Check sheet for the modelled part. Datum: model origin and axes. Units: mm. A direction names the side the tool comes from. Round coordinates to 2 decimals unless told otherwise and drop trailing zeros. Loops run counter-clockwise (first coordinate to the right, second up) from the corner with the lowest first, then second, coordinate; pieces in that order, holes last. Notation, with made-up numbers: M 51,79.25 L 107,79.25 A17 ccw 107,95.25 Z; hole C 68,-24.75 d8. An arc over 180 degrees is marked long. One line per question, with ' | ' between items. Start each with the question number.
(1) Section check A-A (y = 0). Record the boundary of the cut face in (x, z).
(2) Tool access check on faces 4 (the face through (7, 0, 6)), 5 (the face through (-6.459, 8.087, 5.972)), 6 (the face through (0, -7, 6)), 7 (the face through (7.282, 7.355, 5.972)). Record the directions out of +Z, -Z, +X, -X, +Y, -Y that give a thin tool (end or side, any length) a straight path to the whole face; none if there is none.
(3) Section check C-C (y = -12). Record the boundary of the cut face in (x, z), and give its area (3 significant figures).
(4) Draft check along Y on faces 1 (the face through (-7.282, -7.355, 5.972)), 2 (the face through (9.5, -0.1, 2)), 3 (the face through (-8.356, 6.108, 5.972)). Enter one of: +Y half, -Y half, draft (parallel to the pull), parting line (faces both ways), or undercut.
(5) Thickness scan on probe 1 along Y at (x, z) = (0, 5); probe 2 along Y at (x, z) = (0, 3); probe 3 along X at (y, z) = (6, 5.5). Record the ranges inside material, lowest first. Write a range as [from, to].
(6) Go/stop test with flat-tipped pins: P1, Ø2, axis at y = 7.5, z = 2.5, coming from the +X side; P2, Ø4.5, axis at x = -12, y = 0, coming from the +Z side; P3, Ø10, axis at x = 10.5, y = 9, coming from the -Z side; P4, Ø2, axis at y = -10, z = 6, coming from the +X side. Record where each tip stops, or that it passes through.
(7) Section check D-D (z = 2.25). Count the separate pieces of the cut face and the enclosed holes in it, and give its area (3 significant figures).
(8) Section check B-B (x = 2). Record the boundary of the cut face in (y, z).
Autodesk Inventor part; units mm, degrees
ref_plane "YZ Plane" through (0, 0, 0) normal (1, 0, 0) x (0, 1, 0)
ref_plane "XZ Plane" through (0, 0, 0) normal (0, 1, 0) x (-1, 0, 0)
ref_plane "XY Plane" through (0, 0, 0) normal (0, 0, 1) x (1, 0, 0)
sketch "Sketch1" plane through (0, 0, 0) normal (0, 0, 1) x (1, 0, 0)
  circle A0 centre (0, 0) radius 16
  circle A1 centre (0, 0) radius 4
  circle A2 centre (12, 0) radius 2.5
  circle A3 centre (0, 12) radius 2.5
  circle A4 centre (-12, 0) radius 2.5
  circle A5 centre (0, -12) radius 2.5
  dimension "d0" = 32
  dimension "d1" = 8
  dimension "d2" = 5
  dimension "d3" = 12
  dimension "d6" = 360
extrude "Extrusion1" add sketch "Sketch1" along normal blind 4 contours A0 | A1
sketch "Sketch3" plane through (0, 0, 4) normal (0, 0, 1) x (1, 0, 0)
  arc A0 (-6.9584, 12.5904) -> (-5.9892, 8.4411) centre (5.202, 13.243) ccw
  arc A1 (-5.9892, 8.4411) -> (-6.8967, 7.7174) centre (0, 0) ccw
  arc A2 (-6.8967, 7.7174) -> (-10.7263, 9.5856) centre (-14.0685, -2.1247) ccw
  arc A3 (-10.7263, 9.5856) -> (-11.7321, 8.3244) centre (0, 0) ccw
  arc A4 (-11.7321, 8.3244) -> (-9.0586, 5.0065) centre (-1.0591, 14.1885) ccw
  arc A5 (-9.0586, 5.0065) -> (-9.5622, 3.9608) centre (0, 0) ccw
  arc A6 (-9.5622, 3.9608) -> (-13.8231, 3.9824) centre (-11.7534, -8.0184) ccw
  arc A7 (-13.8231, 3.9824) -> (-14.1821, 2.4096) centre (0, 0) ccw
  arc A8 (-14.1821, 2.4096) -> (-10.3337, 0.5803) centre (-7.1104, 12.3239) ccw
  arc A9 (-10.3337, 0.5803) -> (-10.3337, -0.5803) centre (0, 0) ccw
  arc A10 (-10.3337, -0.5803) -> (-14.1821, -2.4096) centre (-7.1104, -12.3239) ccw
  arc A11 (-14.1821, -2.4096) -> (-13.8231, -3.9824) centre (0, 0) ccw
  arc A12 (-13.8231, -3.9824) -> (-9.5622, -3.9608) centre (-11.7534, 8.0184) ccw
  arc A13 (-9.5622, -3.9608) -> (-9.0586, -5.0065) centre (0, 0) ccw
  arc A14 (-9.0586, -5.0065) -> (-11.7321, -8.3244) centre (-1.0591, -14.1885) ccw
  arc A15 (-11.7321, -8.3244) -> (-10.7263, -9.5856) centre (0, 0) ccw
  arc A16 (-10.7263, -9.5856) -> (-6.8967, -7.7174) centre (-14.0685, 2.1247) ccw
  arc A17 (-6.8967, -7.7174) -> (-5.9892, -8.4411) centre (0, 0) ccw
  arc A18 (-5.9892, -8.4411) -> (-6.9584, -12.5904) centre (5.202, -13.243) ccw
  arc A19 (-6.9584, -12.5904) -> (-5.505, -13.2903) centre (0, 0) ccw
  arc A20 (-5.505, -13.2903) -> (-2.8652, -9.9455) centre (-13.5971, -4.1898) ccw
  arc A21 (-2.8652, -9.9455) -> (-1.7337, -10.2038) centre (0, 0) ccw
  arc A22 (-1.7337, -10.2038) -> (-0.8066, -14.3627) centre (10.4327, -9.6744) ccw
  arc A23 (-0.8066, -14.3627) -> (0.8066, -14.3627) centre (0, 0) ccw
  arc A24 (0.8066, -14.3627) -> (1.7337, -10.2038) centre (-10.4327, -9.6744) ccw
  arc A25 (1.7337, -10.2038) -> (2.8652, -9.9455) centre (0, 0) ccw
  arc A26 (2.8652, -9.9455) -> (5.505, -13.2903) centre (13.5971, -4.1898) ccw
  arc A27 (5.505, -13.2903) -> (6.9584, -12.5904) centre (0, 0) ccw
  arc A28 (6.9584, -12.5904) -> (5.9892, -8.4411) centre (-5.202, -13.243) ccw
  arc A29 (5.9892, -8.4411) -> (6.8967, -7.7174) centre (0, 0) ccw
  arc A30 (6.8967, -7.7174) -> (10.7263, -9.5856) centre (14.0685, 2.1247) ccw
  arc A31 (10.7263, -9.5856) -> (11.7321, -8.3244) centre (0, 0) ccw
  arc A32 (11.7321, -8.3244) -> (9.0586, -5.0065) centre (1.0591, -14.1885) ccw
  arc A33 (9.0586, -5.0065) -> (9.5622, -3.9608) centre (0, 0) ccw
  arc A34 (9.5622, -3.9608) -> (13.8231, -3.9824) centre (11.7534, 8.0184) ccw
  arc A35 (13.8231, -3.9824) -> (14.1821, -2.4096) centre (0, 0) ccw
  arc A36 (14.1821, -2.4096) -> (10.3337, -0.5803) centre (7.1104, -12.3239) ccw
  arc A37 (10.3337, -0.5803) -> (10.3337, 0.5803) centre (0, 0) ccw
  arc A38 (10.3337, 0.5803) -> (14.1821, 2.4096) centre (7.1104, 12.3239) ccw
  arc A39 (14.1821, 2.4096) -> (13.8231, 3.9824) centre (0, 0) ccw
  arc A40 (13.8231, 3.9824) -> (9.5622, 3.9608) centre (11.7534, -8.0184) ccw
  arc A41 (9.5622, 3.9608) -> (9.0586, 5.0065) centre (0, 0) ccw
  arc A42 (9.0586, 5.0065) -> (11.7321, 8.3244) centre (1.0591, 14.1885) ccw
  arc A43 (11.7321, 8.3244) -> (10.7263, 9.5856) centre (0, 0) ccw
  arc A44 (10.7263, 9.5856) -> (6.8967, 7.7174) centre (14.0685, -2.1247) ccw
  arc A45 (6.8967, 7.7174) -> (5.9892, 8.4411) centre (0, 0) ccw
  arc A46 (5.9892, 8.4411) -> (6.9584, 12.5904) centre (-5.202, 13.243) ccw
  arc A47 (6.9584, 12.5904) -> (5.505, 13.2903) centre (0, 0) ccw
  arc A48 (5.505, 13.2903) -> (2.8652, 9.9455) centre (13.5971, 4.1898) ccw
  arc A49 (2.8652, 9.9455) -> (1.7337, 10.2038) centre (0, 0) ccw
  arc A50 (1.7337, 10.2038) -> (0.8066, 14.3627) centre (-10.4327, 9.6744) ccw
  arc A51 (0.8066, 14.3627) -> (-0.8066, 14.3627) centre (0, 0) ccw
  arc A52 (-0.8066, 14.3627) -> (-1.7337, 10.2038) centre (10.4327, 9.6744) ccw
  arc A53 (-1.7337, 10.2038) -> (-2.8652, 9.9455) centre (0, 0) ccw
  arc A54 (-2.8652, 9.9455) -> (-5.505, 13.2903) centre (-13.5971, 4.1898) ccw
  arc A55 (-5.505, 13.2903) -> (-6.9584, 12.5904) centre (0, 0) ccw
extrude "Extrusion3" add sketch "Sketch3" along normal blind 4
sketch "Sketch2" plane through (0, 0, 4) normal (0, 0, 1) x (1, 0, 0)
  circle A0 centre (12, 0) radius 2.5
  arc A1 (-1.7381, -10.203) -> (1.7381, -10.203) centre (0, -12) ccw
  arc A2 (1.7381, 10.203) -> (-1.7381, 10.203) centre (0, 12) ccw
  arc A3 (13.5312, -1.9762) -> (13.5312, 1.9762) centre (12, 0) ccw
  circle A4 centre (0, 0) radius 16 construction
  circle A5 centre (12, 0) radius 4.5
  circle A6 centre (0, 12) radius 4.5
  circle A7 centre (-12, 0) radius 4.5
  circle A8 centre (0, -12) radius 4.5
  arc A9 (14.1821, -2.4096) -> (13.5312, -1.9762) centre (7.1104, -12.3239) ccw
  arc A10 (13.8231, -3.9824) -> (14.1821, -2.4096) centre (0, 0) ccw
  arc A11 (9.5622, -3.9608) -> (13.8231, -3.9824) centre (11.7534, 8.0184) ccw
  arc A12 (9.0586, -5.0065) -> (9.5622, -3.9608) centre (0, 0) ccw
  arc A13 (11.7321, -8.3244) -> (9.0586, -5.0065) centre (1.0591, -14.1885) ccw
  arc A14 (10.7263, -9.5856) -> (11.7321, -8.3244) centre (0, 0) ccw
  arc A15 (6.8967, -7.7174) -> (10.7263, -9.5856) centre (14.0685, 2.1247) ccw
  arc A16 (5.9892, -8.4411) -> (6.8967, -7.7174) centre (0, 0) ccw
  arc A17 (6.9584, -12.5904) -> (5.9892, -8.4411) centre (-5.202, -13.243) ccw
  arc A18 (5.505, -13.2903) -> (6.9584, -12.5904) centre (0, 0) ccw
  arc A19 (2.8652, -9.9455) -> (5.505, -13.2903) centre (13.5971, -4.1898) ccw
  arc A20 (1.7381, -10.203) -> (2.8652, -9.9455) centre (0, 0) ccw
  arc A21 (-2.8652, -9.9455) -> (-1.7381, -10.203) centre (0, 0) ccw
  arc A22 (-5.505, -13.2903) -> (-2.8652, -9.9455) centre (-13.5971, -4.1898) ccw
  arc A23 (-6.9584, -12.5904) -> (-5.505, -13.2903) centre (0, 0) ccw
  arc A24 (-5.9892, -8.4411) -> (-6.9584, -12.5904) centre (5.202, -13.243) ccw
  arc A25 (-6.8967, -7.7174) -> (-5.9892, -8.4411) centre (0, 0) ccw
  arc A26 (-10.7263, -9.5856) -> (-6.8967, -7.7174) centre (-14.0685, 2.1247) ccw
  arc A27 (-11.7321, -8.3244) -> (-10.7263, -9.5856) centre (0, 0) ccw
  arc A28 (-9.0586, -5.0065) -> (-11.7321, -8.3244) centre (-1.0591, -14.1885) ccw
  arc A29 (-9.5622, -3.9608) -> (-9.0586, -5.0065) centre (0, 0) ccw
  arc A30 (-13.8231, -3.9824) -> (-9.5622, -3.9608) centre (-11.7534, 8.0184) ccw
  arc A31 (-14.1821, -2.4096) -> (-13.8231, -3.9824) centre (0, 0) ccw
  arc A32 (-13.5312, -1.9762) -> (-14.1821, -2.4096) centre (-7.1104, -12.3239) ccw
  arc A33 (-13.5312, 1.9762) -> (-13.5312, -1.9762) centre (-12, 0) ccw
  arc A34 (-14.1821, 2.4096) -> (-13.5312, 1.9762) centre (-7.1104, 12.3239) ccw
  arc A35 (-13.8231, 3.9824) -> (-14.1821, 2.4096) centre (0, 0) ccw
  arc A36 (-9.5622, 3.9608) -> (-13.8231, 3.9824) centre (-11.7534, -8.0184) ccw
  arc A37 (-9.0586, 5.0065) -> (-9.5622, 3.9608) centre (0, 0) ccw
  arc A38 (-11.7321, 8.3244) -> (-9.0586, 5.0065) centre (-1.0591, 14.1885) ccw
  arc A39 (-10.7263, 9.5856) -> (-11.7321, 8.3244) centre (0, 0) ccw
  arc A40 (-6.8967, 7.7174) -> (-10.7263, 9.5856) centre (-14.0685, -2.1247) ccw
  arc A41 (-5.9892, 8.4411) -> (-6.8967, 7.7174) centre (0, 0) ccw
  arc A42 (-6.9584, 12.5904) -> (-5.9892, 8.4411) centre (5.202, 13.243) ccw
  arc A43 (-5.505, 13.2903) -> (-6.9584, 12.5904) centre (0, 0) ccw
  arc A44 (-2.8652, 9.9455) -> (-5.505, 13.2903) centre (-13.5971, 4.1898) ccw
  arc A45 (-1.7381, 10.203) -> (-2.8652, 9.9455) centre (0, 0) ccw
  arc A46 (2.8652, 9.9455) -> (1.7381, 10.203) centre (0, 0) ccw
  arc A47 (5.505, 13.2903) -> (2.8652, 9.9455) centre (13.5971, 4.1898) ccw
  arc A48 (6.9584, 12.5904) -> (5.505, 13.2903) centre (0, 0) ccw
  arc A49 (5.9892, 8.4411) -> (6.9584, 12.5904) centre (-5.202, 13.243) ccw
  arc A50 (6.8967, 7.7174) -> (5.9892, 8.4411) centre (0, 0) ccw
  arc A51 (10.7263, 9.5856) -> (6.8967, 7.7174) centre (14.0685, -2.1247) ccw
  arc A52 (11.7321, 8.3244) -> (10.7263, 9.5856) centre (0, 0) ccw
  arc A53 (9.0586, 5.0065) -> (11.7321, 8.3244) centre (1.0591, 14.1885) ccw
  arc A54 (9.5622, 3.9608) -> (9.0586, 5.0065) centre (0, 0) ccw
  arc A55 (13.8231, 3.9824) -> (9.5622, 3.9608) centre (11.7534, -8.0184) ccw
  arc A56 (14.1821, 2.4096) -> (13.8231, 3.9824) centre (0, 0) ccw
  arc A57 (13.5312, 1.9762) -> (14.1821, 2.4096) centre (7.1104, 12.3239) ccw
  dimension "d10" = 9
  dimension "d13" = 360
extrude "Extrusion4" cut sketch "Sketch2" along normal blind 4 contours A0 | A0 A57 A56 A55 A5 A11 A10 A9 | A0 A9 A10 A11 A5 A55 A56 A57 | A47 A46 A2 A45 A44 A6 | A6 A44 A45 A2 A46 A47 | A19 A20 A1 A21 A22 A8 | A8 A22 A21 A1 A20 A19 | A36 A35 A34 A33 A32 A31 A30 A7 | A7 A30 A31 A32 A33 A34 A35 A36
sketch "Sketch4" plane through (0, 0, 8) normal (0, 0, 1) x (1, 0, 0)
  circle A0 centre (5, 0) radius 0.85
  circle A1 centre (0, 5) radius 0.85
  circle A2 centre (-5, 0) radius 0.85
  circle A3 centre (0, -5) radius 0.85
  circle A4 centre (5.6569, 5.6569) radius 0.85
  line L0 (0, 0) -> (5.6569, 5.6569) construction
  line L1 (0, 0) -> (5, 0) construction
  circle A5 centre (-5.6569, 5.6569) radius 0.85
  circle A6 centre (-5.6569, -5.6569) radius 0.85
  circle A7 centre (5.6569, -5.6569) radius 0.85
  circle A8 centre (0, 0) radius 0.85
  dimension "d21" = 1.7
  dimension "d22" = 5
  dimension "d25" = 360
  dimension "d27" = 1.7
  dimension "d28" = 45
  dimension "d29" = 8
  dimension "d32" = 360
  dimension "d34" = 1.7
extrude "Extrusion5" cut sketch "Sketch4" against normal through all
sketch "Sketch5" plane through (0, 0, 4) normal (0, 0, 1) x (1, 0, 0)
  circle A0 centre (0, 0) radius 0.85
  arc A1 (-5.9892, 8.4411) -> (-6.8967, 7.7174) centre (0, 0) ccw
  circle A2 centre (0, 0) radius 10.35
  circle A3 centre (0, 0) radius 16
extrude "Extrusion6" cut sketch "Sketch5" along normal through all contours A3
sketch "Sketch6" plane through (0, 0, 4) normal (0, 0, 1) x (1, 0, 0)
  circle A0 centre (12, 0) radius 2.5
  circle A1 centre (12, 0) radius 5
  circle A2 centre (0, 12) radius 5
  circle A3 centre (-12, 0) radius 5
  circle A4 centre (0, -12) radius 5
  point P0 (0, 0)
  dimension "d39" = 10
  dimension "d42" = 360
extrude "Extrusion7" cut sketch "Sketch6" along normal through all contours A0 | A1 | A2 | A3 | A4
properties part number "AC08" material "ABS Plastic"
The answers:
1) outline: M -16,0 L -14.5,0 L -14.5,4 L -16,4 Z; M -9.5,0 L -5.85,0 L -5.85,8 L -7,8 L -7,4 L -9.5,4 Z; M -4.15,0 L -0.85,0 L -0.85,8 L -4.15,8 Z; M 0.85,0 L 4.15,0 L 4.15,8 L 0.85,8 Z; M 5.85,0 L 9.5,0 L 9.5,4 L 7,4 L 7,8 L 5.85,8 Z; M 14.5,0 L 16,0 L 16,4 L 14.5,4 Z
2) face 4: +Z, +X | face 5: +Z, -X, +Y | face 6: +Z, -Y | face 7: +Z, +X, +Y
3) outline: M -10.58,0 L -2.5,0 L -2.5,4 L -10.58,4 Z; M 2.5,0 L 10.58,0 L 10.58,4 L 2.5,4 Z | area: 64.7 mm²
4) face 1: -Y half | face 2: undercut | face 3: +Y half
5) probe 1: [-7, -5.85], [-4.15, -0.85], [0.85, 4.15], [5.85, 7] | probe 2: [-16, -14.5], [-9.5, -5.85], [-4.15, -0.85], [0.85, 4.15], [5.85, 9.5], [14.5, 16] | probe 3: [-8.43, -6.43], [-4.88, 4.88], [6.43, 8.43]
6) P1: x = 14.62 | P2: through | P3: z = 0 | P4: x = 5.11
7) separate pieces: 1 | enclosed holes: 13 | area: 705 mm²
8) outline: M -15.87,0 L -13.5,0 L -13.5,4 L -15.87,4 Z; M -10.5,0 L 10.5,0 L 10.5,4 L 7.42,4 L 7.42,8 L -7.42,8 L -7.42,4 L -10.5,4 Z; M 13.5,0 L 15.87,0 L 15.87,4 L 13.5,4 Z
